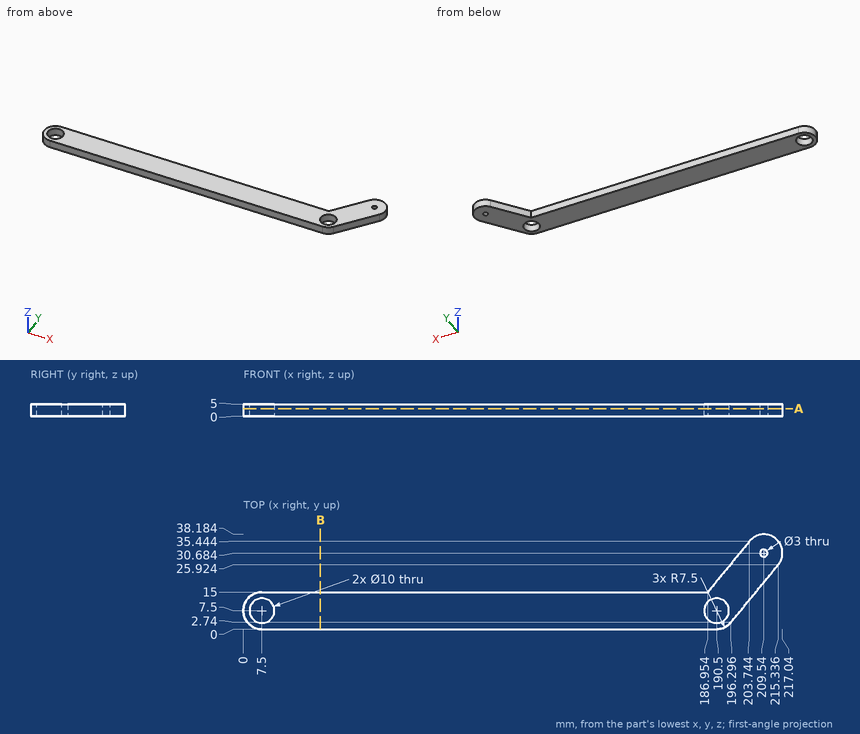
Can you work these out from the drawing? Everything is in mm from the part's minimum corner. Coordinates: 2 decimals unless noted, no trailing zeros. Loops run counter-clockwise (first coordinate to the right, second up) from the corner with the lowest first, then second, coordinate; pieces in that order, holes last. Notation, with made-up numbers: (-3, -31.75) -> (55, -31.75) arc R10 ccw to (55, -27.75) -> close; hole circle Ø9 at (42, 79.25). An arc over 180 degrees is marked (long way). Return JSON: item names as keys, results as strings.
1) Will these pins go through, and if not, where does the flat tip stop? pin 1 (2.5 mm diameter, centred on x = 68, z = 2, fed in from +Y); pin 2 (3 mm diameter, centred on y = 34, z = 3, fed in from -X); pin 3 (3 mm diameter, centred on y = 34.5, z = 2.5, fed in from -X).
Results below:
{"pin 1": "y = 15", "pin 2": "x = 201.33", "pin 3": "x = 201.74"}
2) I need wall thicknesses on line 1 (Y direction, x = 7.5, z = 3.65); line 2 (X direction, y = 4.5, z = 1.4) (1 decimal); line 3 (Y direction, x = 178, z = 2.15). Which ranges of each line are inside material? Lowest first, please. Write a range as from..to.
Results below:
{"line 1": "0..2.5, 12.5..15", "line 2": "0.6..3.5, 11.5..186.5, 194.5..197.7", "line 3": "0..15"}
3) If we section it at A-A, the plane z = 3.1: Write out the boundary of the cut face in (x, y) (1 decimal), then the cut area to 3 significant figures.
Results below:
{"outline": "(7.5, 0) -> (190.5, 0) arc R7.5 ccw to (196.3, 2.7) -> (215.3, 25.9) arc R7.5 ccw to (203.7, 35.4) -> (187, 15) -> (7.5, 15) arc R7.5 ccw to start; hole circle Ø10 at (7.5, 7.5); hole circle Ø10 at (190.5, 7.5); hole circle Ø3 at (209.5, 30.7)", "area": "3,210 mm²"}
4) If we section it at B-B, the plane x = 31: Write out the boundary of the cut face in (y, z).
Results below:
{"outline": "(0, 0) -> (15, 0) -> (15, 5) -> (0, 5) -> close"}
